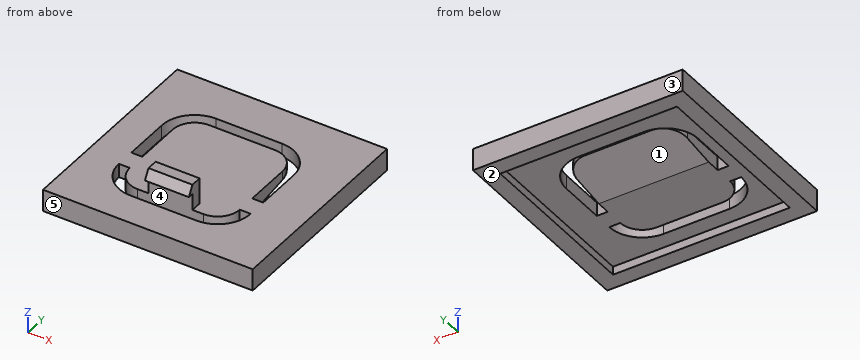
from build123d import *

# Parameters (mm, degrees)
F0_W        = 38.181103766
F0_H        = 37.5636257231
F1_DEPTH    = 2.5
F2_W        = 38.181103766
F2_H        = 37.5636257231
F2_W_2      = 32.181103766
F2_H_2      = 31.5636257231
F3_DEPTH    = 1.5
F5_DEPTH    = 22
F6_DEPTH    = 14
F7_T4_DEPTH = 63.9787194011


# Not quite as in the source:
# - a fillet or chamfer that OpenCascade refuses, or shapes differently, is made with other operations: its cross-section is extruded or revolved along the edge and cut away or added


with BuildPart() as f1:
    # F0 (on Top) → F1 (new body)
    with BuildSketch(Plane.XY):
        with Locations((19.090551883, 18.7818128616)):
            Rectangle(F0_W, F0_H)
        with BuildLine():
            ThreePointArc((8, 12), (9.1715728753, 9.1715728753), (12, 8))
            Line((12, 8), (24, 8))
            ThreePointArc((24, 8), (26.8284271247, 9.1715728753), (28, 12))
            Line((28, 12), (30, 12))
            ThreePointArc((30, 12), (28.2426406871, 7.7573593129), (24, 6))
            Line((24, 6), (12, 6))
            ThreePointArc((12, 6), (7.7573593129, 7.7573593129), (6, 12))
            Line((6, 12), (8, 12))
        make_face(mode=Mode.SUBTRACT)
        with BuildLine():
            Line((24, 28), (12, 28))
            ThreePointArc((12, 28), (9.1715728753, 26.8284271247), (8, 24))
            Line((8, 24), (8, 15.5))
            Line((8, 15.5), (6, 15.5))
            Line((6, 15.5), (6, 24))
            ThreePointArc((6, 24), (7.7573593129, 28.2426406871), (12, 30))
            Line((12, 30), (24, 30))
            ThreePointArc((24, 30), (28.2426406871, 28.2426406871), (30, 24))
            Line((30, 24), (30, 15.5))
            Line((30, 15.5), (28, 15.5))
            Line((28, 15.5), (28, 24))
            ThreePointArc((28, 24), (26.8284271247, 26.8284271247), (24, 28))
        make_face(mode=Mode.SUBTRACT)
    extrude(amount=F1_DEPTH)

    # F2 (on face) → F3 (join)
    with BuildSketch(Plane(origin=(0, 0, 0), x_dir=(1, 0, 0), z_dir=(0, 0, -1))):
        with Locations((19.090551883, -18.7818128616)):
            Rectangle(F2_W, F2_H)
        with Locations((19.090551883, -18.7818128616)):
            Rectangle(F2_W_2, F2_H_2, mode=Mode.SUBTRACT)
    extrude(amount=F3_DEPTH)

    # F4 (on Right) → F5 (join)
    with BuildSketch(Plane.YZ):
        Polygon((8, 5.5), (8, 2.5), (10, 2.5), (10, 7.2320508076), (8, 7.2320508076), (7, 5.5), align=None)
    extrude(amount=F5_DEPTH)

    # F4 (on Right) → F6 (cut)
    with BuildSketch(Plane.YZ):
        Polygon((8, 5.5), (8, 2.5), (10, 2.5), (10, 7.2320508076), (8, 7.2320508076), (7, 5.5), align=None)
    extrude(amount=F6_DEPTH, mode=Mode.SUBTRACT)

    # F7: chamfer of 10 x 1.5 on 1 edges, made by hand


with BuildPart() as f7_tool2:
    # F7_s3 → F7_t4 (new body)
    with BuildSketch(Plane.YZ.offset(49.9893597005)):
        Polygon((18, 0), (28, 1.5), (28, 0), align=None)
    extrude(amount=-F7_T4_DEPTH)

    split(bisect_by=Plane.YZ.offset(8), keep=Keep.TOP)

    split(bisect_by=Plane.YZ.offset(28), keep=Keep.BOTTOM)


with BuildPart() as f1_1:
    add(f1.part)

    # F7_t1: cut F7_tool2
    add(f7_tool2.part, mode=Mode.SUBTRACT)


solid = f1_1.part
Can you work these out from the model? Positions are in its coordinate system, mm. Face numbers are marked on the shaded views. A direction names the side the tool comes from. Round coordinates to 2 decimals unless told otherwise and drop trailing zeros. Loops run counter-clockwise (first coordinate to the right, second up) from the corner with the lowest first, then second, coordinate; pieces in that order, holes last. Notation, with made-up numbers: (-1.75, 30.5) - (12.25, 30.5) arc R16 cw to (12.25, 42.5) - close; hole circle Ø5 at (45, 31). An arc over 180 degrees is marked (long way). Write item = value, one per line. Start each with the question number.
(1) For P1, Ø2, axis at x = 20, y = 5, coming from the -Z side; P2, Ø0.9, axis at y = 8.5, z = 5.5, coming from the +X side; P3, Ø2, axis at x = 24, y = 30, coming from the +Z side, each with a flat end and sliding along its axis, tell me the tip position at first contact or that it passes through.
(2) If we section it at D-D (x = 31): Please give me the cut outline in (y, z).
(3) If we section it at B-B (y = 19): Please give me the cut outline in (x, z).
(4) If we mould it in two halves opening along Y, with no side actions, what happens to the marked faces 3, 4 and 5? For each: released by +Y, released by -Y, zero draft, split by the parting line, or undercut.
(5) If I drill on probe 1 along X at (y, z) = (19, -1); probe 2 along Y at (x, z) = (18, -0.75); probe 3 along Z at (x, y) = (17, 18), over which ranges is the centre line in solid material (lowest first)? Write a range as [from, to].
(6) For the marked faces 1 and 2, which set-ups out of +Z, -Z, +X, -X, +Y, -Y let a thin tool reach every point of the face, with its end or its side?
(7) If we section it at A-A (x = 19.5): Please give me the cut outline in (y, z).
(8) If we section it at C-C (y = 33): Please give me the cut outline in (x, z), and give its area (3 significant figures).
Ans:
q1.P1 = 0
q1.P2 = 22
q1.P3 = 2.5
q2.outline = (0, -1.5) - (3, -1.5) - (3, 0) - (34.56, 0) - (34.56, -1.5) - (37.56, -1.5) - (37.56, 2.5) - (0, 2.5) - close
q3.outline = (0, -1.5) - (3, -1.5) - (3, 0) - (6, 0) - (6, 2.5) - (0, 2.5) - close; (8, 0.15) - (28, 0.15) - (28, 2.5) - (8, 2.5) - close; (30, 0) - (35.18, 0) - (35.18, -1.5) - (38.18, -1.5) - (38.18, 2.5) - (30, 2.5) - close
q4.face_3 = released by +Y
q4.face_4 = undercut
q4.face_5 = released by -Y
q5.probe_1 = [0, 3], [35.18, 38.18]
q5.probe_2 = [0, 3], [34.56, 37.56]
q5.probe_3 = [0, 2.5]
q6.face_1 = -Z
q6.face_2 = -Z, +X, -X, +Y, -Y
q7.outline = (0, -1.5) - (3, -1.5) - (3, 0) - (6, 0) - (6, 2.5) - (0, 2.5) - close; (7, 5.5) - (8, 5.5) - (8, 0) - (18, 0) - (28, 1.5) - (28, 2.5) - (10, 2.5) - (10, 7.23) - (8, 7.23) - close; (30, 0) - (34.56, 0) - (34.56, -1.5) - (37.56, -1.5) - (37.56, 2.5) - (30, 2.5) - close
q8.outline = (0, -1.5) - (3, -1.5) - (3, 0) - (35.18, 0) - (35.18, -1.5) - (38.18, -1.5) - (38.18, 2.5) - (0, 2.5) - close
q8.area = 104 mm²
